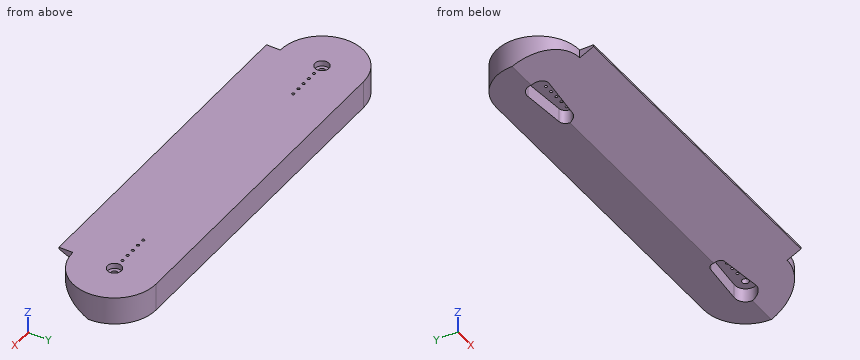
```python
from build123d import *

# Parameters (mm, degrees)
BOSS_EXTRUDE1_DEPTH = 10
CUT_EXTRUDE1_DEPTH  = 5
SKETCH3_R           = 0.5
SKETCH3_R_2         = 1.25
CUT_EXTRUDE2_DEPTH  = 5
SKETCH5_R           = 2.5
CUT_EXTRUDE3_DEPTH  = 2
CHAMFER1_SIZE       = 20
CHAMFER1_SIZE_2     = 9.326153163


with BuildPart() as part:
    # Sketch1 → Boss-Extrude1 (new body)
    with BuildSketch(Plane.XY):
        with BuildLine():
            Line((0, 15), (120, 15))
            ThreePointArc((120, 15), (135, 0), (120, -15))
            Line((120, -15), (120, -20))
            Line((120, -20), (0, -20))
            Line((0, -20), (0, -15))
            ThreePointArc((0, -15), (-15, 0), (0, 15))
        make_face()
    extrude(amount=BOSS_EXTRUDE1_DEPTH)

    # Sketch2 → Cut-Extrude1 (cut)
    with BuildSketch(Plane(origin=(0, 0, 0), x_dir=(-1, 0, 0), z_dir=(0, 0, -1))):
        with BuildLine():
            Line((-119.664370079, 3.860437482), (-103.908464567, 2.490604827))
            ThreePointArc((-103.908464567, 2.490604827), (-101.625, 0), (-103.908464567, -2.490604827))
            Line((-103.908464567, -2.490604827), (-119.664370079, -3.860437482))
            ThreePointArc((-119.664370079, -3.860437482), (-123.875, 0), (-119.664370079, 3.860437482))
        make_face()
    cut_extrude1 = extrude(amount=-CUT_EXTRUDE1_DEPTH, mode=Mode.SUBTRACT)

    # Sketch3 → Cut-Extrude2 (cut)
    with BuildSketch(Plane(origin=(0, 0, 5), x_dir=(-1, 0, 0), z_dir=(0, 0, -1))):
        with Locations((-115.375, 0)):
            Circle(SKETCH3_R)
        with Locations((-112.375, 0)):
            Circle(SKETCH3_R)
        with Locations((-109.375, 0)):
            Circle(SKETCH3_R)
        with Locations((-106.375, 0)):
            Circle(SKETCH3_R)
        with Locations((-103.375, 0)):
            Circle(SKETCH3_R)
        with Locations((-120, 0)):
            Circle(SKETCH3_R_2)
    cut_extrude2 = extrude(amount=-CUT_EXTRUDE2_DEPTH, mode=Mode.SUBTRACT)

    # Sketch5 → Cut-Extrude3 (cut)
    with BuildSketch(Plane.XY.offset(10)):
        with Locations((120, 0)):
            Circle(SKETCH5_R)
    cut_extrude3 = extrude(amount=-CUT_EXTRUDE3_DEPTH, mode=Mode.SUBTRACT)

    # Mirror1: Cut-Extrude1, Cut-Extrude2, Cut-Extrude3 across plane
    add(cut_extrude1.mirror(Plane(origin=(60, 0, 0), x_dir=(0, 0, 1), z_dir=(1, 0, 0))), mode=Mode.SUBTRACT)
    add(cut_extrude2.mirror(Plane(origin=(60, 0, 0), x_dir=(0, 0, 1), z_dir=(1, 0, 0))), mode=Mode.SUBTRACT)
    add(cut_extrude3.mirror(Plane(origin=(60, 0, 0), x_dir=(0, 0, 1), z_dir=(1, 0, 0))), mode=Mode.SUBTRACT)

    # Chamfer1
    # the kernel refuses this chamfer: 20, 9.326153163 mm, written as the material it takes off along each edge
    with BuildSketch(Plane(origin=(171.819509428, -20, 0), x_dir=(0, 0.9998669641130704, -0.016311164131110348), z_dir=(-1, 0, 0))) as chamfer1_piece_1:
        Polygon((CHAMFER1_SIZE * 0.999866964113, -CHAMFER1_SIZE * 0.0163111641311), (-CHAMFER1_SIZE_2 * 0.0163111641313, -CHAMFER1_SIZE_2 * 0.999866964124), (0, 0), align=None)
    extrude(amount=223.639018857, mode=Mode.SUBTRACT)


solid = part.part
```
Verification items for the finished model (mm, model axes). Round coordinates to 2 decimals unless told otherwise and drop trailing zeros. Order: outer loops, then holes, each group sorted by start corner. A loop starts at its lowest first (then second) coordinate and runs counter-clockwise, first axis right, second up.
1) Depth check by flat-ended pin: pin 1 (7 mm diameter, centred on x = 0, y = 0, fed in from -Z); pin 2 (1.5 mm diameter, centred on x = 119.5, y = -1, fed in from +Z); pin 3 (2 mm diameter, centred on x = 34, z = 3.5, fed in from -Y). Enter the tip coordinate at first touch or a pass-through.
Geometry says:
pin 1: stops at z = 5
pin 2: stops at z = 8
pin 3: stops at y = -9.65
2) Cross-section at D-D, the plane y = -11. Record the cut outline in (x, z), plus the area to 3 significant figures.
Geometry says:
outline: (-10.2, 5.13) - (130.2, 5.13) - (130.2, 10) - (-10.2, 10) - close
area: 684 mm2
3) Material ranges on line 1 (X direction, y = -1, z = 8.75); line 2 (Y direction, x = 67, z = 6.5); line 3 (Z direction, x = 96, y = -13.5), recorded low to high.
Geometry says:
line 1: x = -14.97 to -2.29, 2.29 to 117.71, 122.29 to 134.97
line 2: y = -13.94 to 15
line 3: z = 6.3 to 10
4) Cross-section at B-B, the plane z = 3.25. Record the cut outline in (x, y) (3 decimals), plus the area to 3 significant figures.
Geometry says:
outline: (-13.282, -6.97) - (133.282, -6.97) arc R15 ccw to (120, 15) - (0, 15) arc R15 ccw to start; hole (0.336, -3.86) - (16.092, -2.491) arc R2.5 ccw to (16.092, 2.491) - (0.336, 3.86) arc R3.875 ccw (long way) to start; hole (103.908, -2.491) - (119.664, -3.86) arc R3.875 ccw (long way) to (119.664, 3.86) - (103.908, 2.491) arc R2.5 ccw to start
area: 2,920 mm2
5) Cross-section at A-A, the plane x = 70. Record the cut outline in (y, z), plus the area to 3 significant figures.
Geometry says:
outline: (-20, 9.33) - (0, 0) - (15, 0) - (15, 10) - (-20, 10) - close
area: 257 mm2
6) Cross-section at C-C, the plane y = 8. Record the cut outline in (x, z), plus the area to 3 significant figures.
Geometry says:
outline: (-12.69, 0) - (132.69, 0) - (132.69, 10) - (-12.69, 10) - close
area: 1,450 mm2
